Part model, mm, in its own coordinate system. Round coordinates to 2 decimals unless told otherwise and drop trailing zeros. Order: outer loops, then holes, each group sorted by start corner. A loop starts at its lowest first (then second) coordinate and runs counter-clockwise, first axis right, second up. Notation, with made-up numbers: (21.5, 7.25) -> (49.5, 7.25) arc R35 ccw to (49.5, 46.25) -> close; hole circle Ø1 at (-18.5, -16.5). An arc over 180 degrees is marked (long way). Use CSV: the item, a comma, the result in double quotes.
```python
from build123d import *

# Parameters (mm, degrees)
SKETCH1_W                    = 80
SKETCH1_H                    = 60
SKETCH1_R                    = 3.1
SKETCH1_R_2                  = 3.25
BOSS_EXTRUDE1_DEPTH          = 6.35
FILLET1_R                    = 10
CSK_FOR_M6_SFHCS1_AT_2_COUNT = 2
CSK_FOR_M6_SFHCS1_AT_2_PITCH = 20
CSK_FOR_M6_SFHCS1_AT_3_COUNT = 2
CSK_FOR_M6_SFHCS1_AT_3_PITCH = 40


with BuildPart() as part:
    # Sketch1 → Boss-Extrude1 (new body)
    with BuildSketch(Plane(origin=(0, 0, 0), x_dir=(1, 0, 0), z_dir=(0, 1, 0))):
        with Locations((40, 30)):
            Rectangle(SKETCH1_W, SKETCH1_H)
        with Locations((40, 7.5)):
            Circle(SKETCH1_R, mode=Mode.SUBTRACT)
        with Locations((20, 7.5)):
            Circle(SKETCH1_R, mode=Mode.SUBTRACT)
        with Locations((60, 7.5)):
            Circle(SKETCH1_R, mode=Mode.SUBTRACT)
        with Locations((35, 52.5)):
            Circle(SKETCH1_R_2, mode=Mode.SUBTRACT)
        with Locations((45, 52.5)):
            Circle(SKETCH1_R_2, mode=Mode.SUBTRACT)
        with Locations((25, 52.5)):
            Circle(SKETCH1_R_2, mode=Mode.SUBTRACT)
        with Locations((30, 42.5)):
            Circle(SKETCH1_R_2, mode=Mode.SUBTRACT)
        with Locations((40, 42.5)):
            Circle(SKETCH1_R_2, mode=Mode.SUBTRACT)
        with Locations((50, 42.5)):
            Circle(SKETCH1_R_2, mode=Mode.SUBTRACT)
        with Locations((20, 42.5)):
            Circle(SKETCH1_R_2, mode=Mode.SUBTRACT)
        with Locations((15, 52.5)):
            Circle(SKETCH1_R_2, mode=Mode.SUBTRACT)
        with Locations((55, 52.5)):
            Circle(SKETCH1_R_2, mode=Mode.SUBTRACT)
        with Locations((65, 52.5)):
            Circle(SKETCH1_R_2, mode=Mode.SUBTRACT)
        with Locations((60, 42.5)):
            Circle(SKETCH1_R_2, mode=Mode.SUBTRACT)
        with Locations((75, 47.5)):
            Circle(SKETCH1_R_2, mode=Mode.SUBTRACT)
        with Locations((5, 47.5)):
            Circle(SKETCH1_R_2, mode=Mode.SUBTRACT)
    extrude(amount=BOSS_EXTRUDE1_DEPTH)

    # Fillet1
    fillet1_edges = [part.edges().sort_by_distance(p)[0] for p in [
        (0, 3.175, 0),
        (0, 3.175, -60),
        (80, 3.175, -60),
        (80, 3.175, 0),
    ]]
    fillet(fillet1_edges, radius=FILLET1_R)

    # Sketch3 → CSK for M6 SFHCS1 (revolve, cut)
    with BuildSketch(Plane(origin=(20, 6.35, -7.5), x_dir=(0, 0, 1), z_dir=(1, 0, 0))):
        Polygon((0, 0), (0, 6.35), (3.3, 6.35), (3.3, 3.42), (6.72, 0), align=None)
    csk_for_m6_sfhcs1 = revolve(axis=Axis((20, 12.7, -7.5), (0, -1, 0)), mode=Mode.SUBTRACT)

    # CSK for M6 SFHCS1 at 2: CSK for M6 SFHCS1 ×2
    with Locations(*[(i * CSK_FOR_M6_SFHCS1_AT_2_PITCH, 0, 0) for i in range(1, CSK_FOR_M6_SFHCS1_AT_2_COUNT)]):
        add(csk_for_m6_sfhcs1, mode=Mode.SUBTRACT)

    # CSK for M6 SFHCS1 at 3: CSK for M6 SFHCS1 ×2
    with Locations(*[(i * CSK_FOR_M6_SFHCS1_AT_3_PITCH, 0, 0) for i in range(1, CSK_FOR_M6_SFHCS1_AT_3_COUNT)]):
        add(csk_for_m6_sfhcs1, mode=Mode.SUBTRACT)


solid = part.part
```
(1) Cut at B-B, the plane z = -47.5. Give the cut face in (x, y).
Reply:
outline,"(0, 0) -> (1.75, 0) -> (1.75, 6.35) -> (0, 6.35) -> close; (8.25, 0) -> (71.75, 0) -> (71.75, 6.35) -> (8.25, 6.35) -> close; (78.25, 0) -> (80, 0) -> (80, 6.35) -> (78.25, 6.35) -> close"
(2) Pull direction Z, two halves, no side cores. Call faces 1 (the face through (2.85, 3.22, -56.99)), 2 (the face through (31.5, 3.131, -39.617)), 3 (the face through (39, 6.35, -30)): released by +Z, released by -Z, zero draft, split by the parting line, or undercut.
Reply:
face 1,"released by -Z"
face 2,"undercut"
face 3,"zero draft"
(3) Cut at C-C, the plane y = 3.75. State how many separate pieces and enclosed holes the cut face has, then the cut area to 3 significant figures.
Reply:
separate pieces,"1"
enclosed holes,"16"
area,"4,120 mm2"
(4) Cut at A-A, the plane x = 40. Give the cut face in (y, z).
Reply:
outline,"(0, -60) -> (6.35, -60) -> (6.35, -45.75) -> (0, -45.75) -> close; (0, -39.25) -> (6.35, -39.25) -> (6.35, -14.22) -> (2.93, -10.8) -> (0, -10.8) -> close; (0, -4.2) -> (2.93, -4.2) -> (6.35, -0.78) -> (6.35, 0) -> (0, 0) -> close"
(5) Cut at D-D, the plane x = 30. Give the cut face in (y, z), then the cut area to 3 significant figures.
Reply:
outline,"(0, -60) -> (6.35, -60) -> (6.35, -45.75) -> (0, -45.75) -> close; (0, -39.25) -> (6.35, -39.25) -> (6.35, 0) -> (0, 0) -> close"
area,"340 mm2"
(6) Drop flat-ended pins along their axis: P1, Ø8.5, axis at x = 25, z = -52.5, coming from the -Y side; P2, Ø6, axis at x = 30, z = -42.5, coming from the -Y side; P3, Ø10.5, axis at x = 60, z = -7.5, coming from the +Y side. Give the stop position or say it passes through.
Reply:
P1,"y = 0"
P2,"through"
P3,"y = 4.88"
(7) Probe probe 1 along Z at (x, y) = (40, 0.8); probe 2 along X at (y, z) = (3.75, -42.5); probe 3 along Z at (x, y) = (57, 0.5). List the from-to ranges inside material, lowest first. Write a range as [from, to].
Reply:
probe 1,"[-60, -45.75], [-39.25, -10.8], [-4.2, 0]"
probe 2,"[0, 16.75], [23.25, 26.75], [33.25, 36.75], [43.25, 46.75], [53.25, 56.75], [63.25, 80]"
probe 3,"[-60, -55.06], [-49.94, -43.75], [-41.25, -8.87], [-6.13, 0]"
